Verification items for the finished model (mm, model axes). A direction names the side the tool comes from. Round coordinates to 2 decimals unless told otherwise and drop trailing zeros. Write each loop counter-clockwise with the first axis right and the second up, starting at its lowest first coordinate (ties: lowest second). Pieces come first, ordered by that corner, then holes. Notation, with made-up numbers: M 73.5,18.5 L 129.5,18.5 A27 ccw 129.5,52.5 Z; hole C 83.5,61.5 d11. An arc over 180 degrees is marked long. One line per item, written item: value. Start each with the question number.
Item 1: Gauge pin test, flat ends, axial feed: pin 1 (1.5 mm diameter, centred on x = -73.5, y = 2.5, fed in from +Z); pin 2 (5.5 mm diameter, centred on x = -140.5, z = 3.5, fed in from +Y); pin 3 (1.5 mm diameter, centred on x = -70, z = -91.5, fed in from -Y). Record the tip position at first contact, or that the pin passes through.
Item 2: Draft check along X on faces 5 (the face through (0, 30, -46)), 6 (the face through (-99, 31, -87)), 7 (the face through (-200, 30, -44)), 8 (the face through (-99, 10, -92)). Enter one of: +X half, -X half, draft (parallel to the pull), parting line (faces both ways), or undercut.
Item 3: Section check B-B, the plane x = -126. Record the cut outline in (y, z), then the cut area to 3 significant figures.
Item 4: Tool access check on faces 1 (the face through (-101, 2, -90)), 2 (the face through (-99, 35, 0)), 3 (the face through (-99, 5, 2)), 4 (the face through (-197, 31, -46)). Record the directions out of +Z, -Z, +X, -X, +Y, -Y that give a thin tool (end or side, any length) a straight path to the whole face; none if there is none.
Item 5: Thickness scan on probe 1 along X at (y, z) = (41, -62); probe 2 along Z at (x, y) = (-29.5, 16.5); probe 3 along Z at (x, y) = (-43, 8.5). Record the ranges inside material, lowest first. Write a range as from..to.
Item 6: Section check A-A, the plane y = 16. Record the cut outline in (x, z).
Item 7: Section check C-C, the plane z = -19.5. Record the cut outline in (x, y).
Item 8: Section check D-D, the plane x = -171.5. Record the cut outline in (y, z), then the cut area to 3 significant figures.
Autodesk Inventor part; units mm, degrees
ref_plane "YZ Plane" through (0, 0, 0) normal (1, 0, 0) x (0, 1, 0)
ref_plane "XZ Plane" through (0, 0, 0) normal (0, 1, 0) x (-1, 0, 0)
ref_plane "XY Plane" through (0, 0, 0) normal (0, 0, 1) x (1, 0, 0)
sketch "Sketch1" plane through (0, 0, 0) normal (0, 1, 0) x (-1, 0, 0)
  line L0 (0, 0) -> (200, 0)
  line L1 (200, 0) -> (200, -90)
  line L2 (200, -90) -> (0, -90)
  line L3 (0, -90) -> (0, 0)
  line L4 (197, -87) -> (197, -3)
  line L5 (197, -3) -> (3, -3)
  line L6 (3, -3) -> (3, -87)
  line L7 (3, -87) -> (197, -87)
  dimension "d0" = 200
  dimension "d1" = 90
  dimension "d2" = 3
extrude "Extrusion1" add sketch "Sketch1" along normal blind 60
sketch "Sketch2" plane through (-200, 0, 0) normal (0, 0, 1) x (1, 0, 0)
  line L0 (0, 0) -> (0, 60)
  line L1 (200, 0) -> (200, 60)
  line L2 (0, 10) -> (200, 10)
  line L3 (200, 10) -> (200, 5)
  line L4 (200, 5) -> (0, 5)
  line L5 (0, 5) -> (0, 10)
  line L6 (0, 0) -> (200, 0)
  point P0 (0, 5)
  dimension "d5" = 5
  dimension "d6" = 5
extrude "Extrusion2" add sketch "Sketch2" along normal blind 5 contours L0 L2 L1 L4
sketch "Sketch3" plane through (0, 0, -90) normal (0, 0, -1) x (-1, 0, 0)
  line L0 (0, 0) -> (0, 60)
  line L1 (200, 0) -> (200, 60)
  line L2 (0, 10) -> (200, 10)
  line L3 (200, 10) -> (200, 5)
  line L4 (200, 5) -> (0, 5)
  line L5 (0, 5) -> (0, 10)
  line L6 (0, 0) -> (200, 0)
  point P0 (0, 5)
  dimension "d9" = 5
  dimension "d10" = 5
extrude "Extrusion3" add sketch "Sketch3" along normal blind 5 contours L0 L2 L1 L4
sketch "Sketch4" plane through (0, 0, 0) normal (0, -1, 0) x (1, 0, 0)
  line L0 (-197, -3) -> (-197, -87)
  line L1 (-3, -3) -> (-197, -3)
  line L2 (-197, -3) -> (-197, -87)
  line L3 (-197, -87) -> (-3, -87)
  line L4 (-3, -87) -> (-3, -3)
  line L5 (-50, -30) -> (-150, -30)
  line L6 (-150, -30) -> (-150, -60)
  line L7 (-150, -60) -> (-50, -60)
  line L8 (-50, -60) -> (-50, -30)
  line L9 (-200, -90) -> (-200, 0)
  line L10 (-200, 0) -> (0, 0)
  dimension "d13" = 100
  dimension "d14" = 30
  dimension "d16" = 50
  dimension "d17" = 30
extrude "Extrusion4" add sketch "Sketch4" against normal blind 3
properties part number "caja de mascarilllas"
Response values:
1. pin 1: stops at z = 0
1. pin 2: stops at y = 10
1. pin 3: stops at y = 5
2. face 5: +X half
2. face 6: undercut
2. face 7: -X half
2. face 8: draft
3. outline: M 0,-90 L 5,-90 L 5,-95 L 10,-95 L 10,-90 L 60,-90 L 60,-87 L 3,-87 L 3,-60 L 0,-60 Z; M 0,-30 L 3,-30 L 3,-3 L 60,-3 L 60,0 L 10,0 L 10,5 L 5,5 L 5,0 L 0,0 Z
3. area: 572 mm2
4. face 1: -Z, +X, -X, -Y
4. face 2: +Z, +X, -X, +Y
4. face 3: +Z, +X, -X, -Y
4. face 4: +Y
5. probe 1: x = -200..-197, -3..0
5. probe 2: z = -90..-87, -3..0
5. probe 3: z = -95..-87, -3..5
6. outline: M -200,-90 L 0,-90 L 0,0 L -200,0 Z; hole M -197,-87 L -3,-87 L -3,-3 L -197,-3 Z
7. outline: M -200,0 L 0,0 L 0,60 L -3,60 L -3,3 L -197,3 L -197,60 L -200,60 Z
8. outline: M 0,-90 L 5,-90 L 5,-95 L 10,-95 L 10,-90 L 60,-90 L 60,-87 L 3,-87 L 3,-3 L 60,-3 L 60,0 L 10,0 L 10,5 L 5,5 L 5,0 L 0,0 Z
8. area: 662 mm2
